from build123d import *

# Parameters (mm, degrees)
F0_W     = 63
F0_H     = 131
F0_W_2   = 12
F0_H_2   = 11
F1_DEPTH = 3
F0_H_3   = 5
F2_DEPTH = 12
F3_R     = 17


with BuildPart() as f1:
    # F0 (on Front) → F1 (new body)
    with BuildSketch(Plane.XZ):
        Rectangle(F0_W, F0_H)
        with Locations((0, 50.5)):
            Rectangle(F0_W_2, F0_H_2, mode=Mode.SUBTRACT)
    extrude(amount=F1_DEPTH)

    # F0 (on Front) → F2 (join)
    with BuildSketch(Plane.XZ):
        Polygon((31.5, -70.5), (36.5, -70.5), (36.5, 70.5), (31.5, 70.5), (31.5, 65.5), (31.5, -65.5), align=None)
        with Locations((0, -68)):
            Rectangle(F0_W, F0_H_3)
        Polygon((-36.5, -70.5), (-31.5, -70.5), (-31.5, -65.5), (-31.5, 65.5), (-31.5, 70.5), (-36.5, 70.5), align=None)
        with Locations((0, 68)):
            Rectangle(F0_W, F0_H_3)
    extrude(amount=F2_DEPTH)

    # F3
    f3_edges = [f1.edges().sort_by_distance(p)[0] for p in [
        (36.5, -6, 70.5),
        (-36.5, -6, 70.5),
        (-36.5, -6, -70.5),
        (36.5, -6, -70.5),
    ]]
    fillet(f3_edges, radius=F3_R)


solid = f1.part
The listing builds one solid part. Answer for the finished solid, in the listing's coordinates (mm). A direction names the side the tool comes from. Round coordinates to 2 decimals unless told otherwise and drop trailing zeros. Write each loop counter-clockwise with the first axis right and the second up, starting at its lowest first coordinate (ties: lowest second). Pieces come first, ordered by that corner, then holes. Notation, with made-up numbers: (39.5, 82) - (92.5, 82) arc R16 cw to (92.5, 104) - close; hole circle Ø1 at (36, 30). An arc over 180 degrees is marked (long way). Use one line per item in the form item = value. Start each with the question number.
Item 1: A cutting plane is placed at D-D (z = -8). Write down the section's boundary in (x, y), plus the area to 3 significant figures.
Item 2: A cutting plane is placed at B-B (y = -7.25). Write down the section's boundary in (x, z).
Item 3: Find the intervals of material crossed by line 1 (X direction, y = -9.25, z = -44); line 2 (Z direction, x = 5, y = -9); line 3 (Z direction, x = 2.5, y = -1.75), in increasing order. Write a range as [from, to].
Item 4: A tool of negligible diameter and unlimited length cuts with its end or side. For faces 1 (the flat face through (0, -7, 65.5)), 2 (the flat face through (-36.5, -6, 1)), 3 (the flat face through (6, -1, 50)), from which of +Z, -Z, +X, -X, +Y, -Y can it reach the whole face along a straight path? Write none if from no direction.
Item 5: A cutting plane is placed at A-A (z = 50). Write down the section's boundary in (x, y), plus the area to 3 significant figures.
Item 6: A cutting plane is placed at C-C (x = -9). Write down the section's boundary in (y, z), plus the area to 3 significant figures.
Item 7: Flat-ended cylindrical pins translate along their axes: pin 1 Ø6 at (x, z) = (-11, -52.5) entering from -Y; pin 2 Ø1 at (y, z) = (-9, 56) entering from +X. Find the tip coordinate at first contact, or state that the pin passes through.
Item 8: Determine the mould class of faces 4 (the flat face through (31.5, -7, 1)), 5 (the flat face through (36.5, -6, -1)), 6 (the flat face through (0, -3, 1)), 7 (the flat face through (0, -6, 70.5)) for opening direction Z: +Z half, -Z half, draft (parallel to the pull), parting line (faces both ways), or undercut.
The answers:
q1.outline = (-36.5, -12) - (-31.5, -12) - (-31.5, -3) - (31.5, -3) - (31.5, -12) - (36.5, -12) - (36.5, 0) - (-36.5, 0) - close
q1.area = 309 mm^2
q2.outline = (-36.5, -53.5) arc R17 ccw to (-19.5, -70.5) - (19.5, -70.5) arc R17 ccw to (36.5, -53.5) - (36.5, 53.5) arc R17 ccw to (19.5, 70.5) - (-19.5, 70.5) arc R17 ccw to (-36.5, 53.5) - close; hole (-31.5, -65.5) - (31.5, -65.5) - (31.5, 65.5) - (-31.5, 65.5) - close
q3.line_1 = [-36.5, -31.5], [31.5, 36.5]
q3.line_2 = [-70.5, -65.5], [65.5, 70.5]
q3.line_3 = [-70.5, 45], [56, 70.5]
q4.face_1 = -Y
q4.face_2 = +Z, -Z, -X, +Y, -Y
q4.face_3 = +Y, -Y
q5.outline = (-36.5, -12) - (-31.5, -12) - (-31.5, -3) - (-6, -3) - (-6, 0) - (-36.5, 0) - close; (6, -3) - (31.5, -3) - (31.5, -12) - (36.5, -12) - (36.5, 0) - (6, 0) - close
q5.area = 273 mm^2
q6.outline = (-12, -70.5) - (0, -70.5) - (0, 70.5) - (-12, 70.5) - (-12, 65.5) - (-3, 65.5) - (-3, -65.5) - (-12, -65.5) - close
q6.area = 513 mm^2
q7.pin_1 = -3
q7.pin_2 = 36.38
q8.face_4 = undercut
q8.face_5 = draft
q8.face_6 = undercut
q8.face_7 = +Z half
